Answer from the drawing. Dimensions are ordinates in mm from the lowest x, y and z of the part. A direction names the side the tool comes from. Give positions to 0.01 mm unless a question says otherwise; leave off trailing zeros. Order: outer loops, then holes, each group sorted by start corner. A loop starts at its lowest first (then second) coordinate and runs counter-clockwise, first axis right, second up. Notation, with made-up numbers: (66, 46.25) - (115, 46.25) arc R25 ccw to (115, 85.25) - close; hole circle Ø5 at (-33.75, 30). An arc over 180 degrees is marked (long way). Answer in a Markdown table with one row per item.
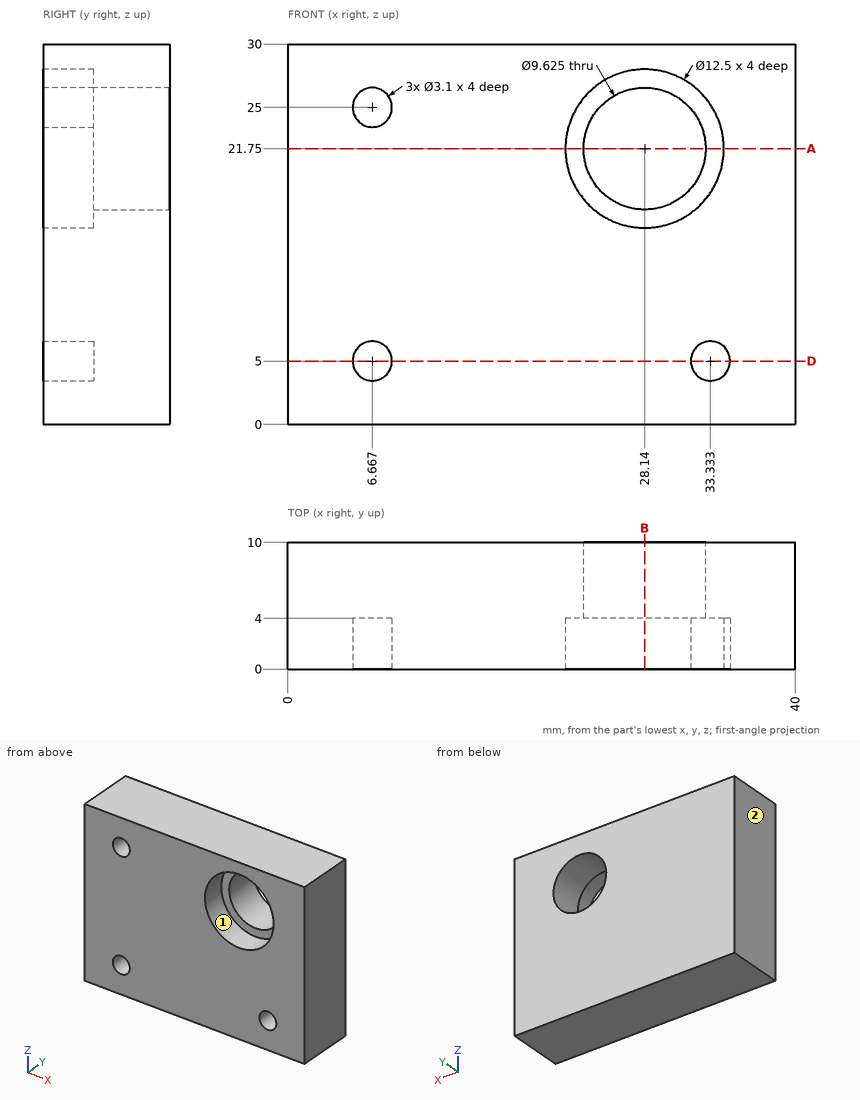
Item 1: This flat-tipped pin is pushed along its axis until it touches: P1, Ø0.9, axis at x = 7, z = 4.5, coming from the -Y side. Where does it stop, or does it pass through?
Answer block:
| item | result |
|---|---|
| P1 | y = 4 |
Item 2: Which of the six approach directions +Z, -Z, +X, -X, +Y, -Y give full straight-line access (tool end or side, diameter ignored) to the marked faces 1 and 2?
Answer block:
| item | result |
|---|---|
| face 1 | -Y |
| face 2 | +Z, -Z, -X, +Y, -Y |
Item 3: Find section A-A on z = 21.75. Write down the section's boundary in (x, y), then the cut area to 3 significant figures.
Answer block:
| item | result |
|---|---|
| outline | (0, 0) - (21.89, 0) - (21.89, 4) - (23.33, 4) - (23.33, 10) - (0, 10) - close; (32.95, 4) - (34.39, 4) - (34.39, 0) - (40, 0) - (40, 10) - (32.95, 10) - close |
| area | 292 mm² |
Item 4: Find section D-D on z = 5. Write down the section's boundary in (x, y).
Answer block:
| item | result |
|---|---|
| outline | (0, 0) - (5.12, 0) - (5.12, 4) - (8.22, 4) - (8.22, 0) - (31.78, 0) - (31.78, 4) - (34.88, 4) - (34.88, 0) - (40, 0) - (40, 10) - (0, 10) - close |
Item 5: Find section B-B on x = 28.14. Write down the section's boundary in (y, z), then the cut area to 3 significant figures.
Answer block:
| item | result |
|---|---|
| outline | (0, 0) - (10, 0) - (10, 16.94) - (4, 16.94) - (4, 15.5) - (0, 15.5) - close; (0, 28) - (4, 28) - (4, 26.56) - (10, 26.56) - (10, 30) - (0, 30) - close |
| area | 192 mm² |
Item 6: Consider line 1 (X direction, y = 2.8, z = 5); line 2 (X direction, y = 8.05, z = 21.75); line 3 (X direction, y = 1, z = 4). Determine where each line is inside the solid, lowest interval first.
Answer block:
| item | result |
|---|---|
| line 1 | 0 to 5.12, 8.22 to 31.78, 34.88 to 40 |
| line 2 | 0 to 23.33, 32.95 to 40 |
| line 3 | 0 to 5.48, 7.85 to 32.15, 34.52 to 40 |
